For this review, take the finished solid that the model builds, in its own axes (mm). Coordinates: 2 decimals unless noted, no trailing zeros. Loops run counter-clockwise (first coordinate to the right, second up) from the corner with the lowest first, then second, coordinate; pieces in that order, holes last. Notation, with made-up numbers: M 65.25,18.25 L 99.25,18.25 A32 ccw 99.25,57.25 Z; hole C 58.5,44 d6. An arc over 180 degrees is marked long. Write each question's results on one line, items separated by ' | '. Start each with the question number.
```python
from build123d import *

# Parameters (mm, degrees)
F0_R     = 2
F1_DEPTH = 2


# Not quite as in the source:
# - a feature names something its author has since deleted; it is built from what else it names


with BuildPart() as f1:
    # F0 (on Top) → F1 (new body)
    with BuildSketch(Plane.XY):
        with BuildLine():
            Line((56.6317902379, -3.0349094544), (56.6317902379, 10.5057977874))
            ThreePointArc((56.6317902379, 10.5057977874), (57.9282334063, 11.0612910292), (58.8036425211, 9.955399302))
            Line((58.8036425211, 9.955399302), (58.8036425211, -3.3060063632))
            ThreePointArc((58.8036425211, -3.3060063632), (58.8059571474, -3.4285186947), (58.8128977225, -3.5508561677))
            Line((58.8128977225, -3.5508561677), (68.3904010917, -2.8257703951))
            ThreePointArc((68.3904010917, -2.8257703951), (69.9985927846, -2.4288509841), (71.3888536722, -1.5282954863))
            Line((71.3888536722, -1.5282954863), (71.9441100955, 13.8000454754))
            ThreePointArc((71.9441100955, 13.8000454754), (70.4479915869, 14.8624188349), (68.6693633039, 15.3135165823))
            Line((68.6693633039, 15.3135165823), (58.6544042145, 15.9537835574))
            Line((58.6544042145, 15.9537835574), (2.6067622363, 15.9537835574))
            ThreePointArc((2.6067622363, 15.9537835574), (0.4614561486, 15.0651686804), (-0.4271587284, 12.9198625927))
            Line((-0.4271587284, 12.9198625927), (-0.4271587284, -3.0349094544))
            Line((-0.4271587284, -3.0349094544), (3.8183579072, -3.0349094544))
            Line((3.8183579072, -3.0349094544), (3.8183579072, 2.3688513962))
            Line((3.8183579072, 2.3688513962), (3.8183579072, 10.5057977874))
            ThreePointArc((3.8183579072, 10.5057977874), (4.9481016159, 11.1006888991), (6.0778453246, 10.5057977874))
            Line((6.0778453246, 10.5057977874), (6.0778453246, 2.3688513962))
            Line((6.0778453246, 2.3688513962), (6.0778453246, -3.0349094544))
            ThreePointArc((6.0778453246, -3.0349094544), (6.9707155924, -3.9277797221), (7.8635858601, -3.0349094544))
            Line((7.8635858601, -3.0349094544), (7.8635858601, 2.3688513962))
            Line((7.8635858601, 2.3688513962), (7.8635858601, 10.5057977874))
            ThreePointArc((7.8635858601, 10.5057977874), (8.8748928484, 11.1003156957), (9.8861998366, 10.5057977874))
            Line((9.8861998366, 10.5057977874), (9.8861998366, 2.3688513962))
            Line((9.8861998366, 2.3688513962), (9.8861998366, -3.0349094544))
            ThreePointArc((9.8861998366, -3.0349094544), (10.8975068249, -4.0462164426), (11.9088138131, -3.0349094544))
            Line((11.9088138131, -3.0349094544), (11.9088138131, 2.3688513962))
            Line((11.9088138131, 2.3688513962), (11.9088138131, 10.5057977874))
            ThreePointArc((11.9088138131, 10.5057977874), (12.9201208014, 11.1003953408), (13.9314277896, 10.5057977874))
            Line((13.9314277896, 10.5057977874), (13.9314277896, 2.3688513962))
            Line((13.9314277896, 2.3688513962), (13.9314277896, -3.0349094544))
            ThreePointArc((13.9314277896, -3.0349094544), (14.9427347779, -4.0462164426), (15.9540417661, -3.0349094544))
            Line((15.9540417661, -3.0349094544), (15.9540417661, 2.3688513962))
            Line((15.9540417661, 2.3688513962), (15.9540417661, 10.5057977874))
            ThreePointArc((15.9540417661, 10.5057977874), (16.9653487543, 11.1012729968), (17.9766557426, 10.5057977874))
            Line((17.9766557426, 10.5057977874), (17.9766557426, -3.0349094544))
            Line((17.9766557426, -3.0349094544), (17.9766557426, -3.0600128507))
            ThreePointArc((17.9766557426, -3.0600128507), (18.987884836, -4.0587681408), (19.9991139294, -3.0600128507))
            Line((19.9991139294, -3.0600128507), (19.9991139294, -3.0349094544))
            Line((19.9991139294, -3.0349094544), (19.9991139294, 2.3688513962))
            Line((19.9991139294, 2.3688513962), (19.9991139294, 10.5057977874))
            ThreePointArc((19.9991139294, 10.5057977874), (21.0104988125, 11.0625593301), (22.0218836956, 10.5057977874))
            Line((22.0218836956, 10.5057977874), (22.0218836956, 2.3688513962))
            Line((22.0218836956, 2.3688513962), (22.0218836956, -3.0349094544))
            ThreePointArc((22.0218836956, -3.0349094544), (23.0331906838, -4.0270898738), (24.0444976721, -3.0349094544))
            Line((24.0444976721, -3.0349094544), (24.0444976721, 2.3688513962))
            Line((24.0444976721, 2.3688513962), (24.0444976721, 10.5057977874))
            ThreePointArc((24.0444976721, 10.5057977874), (25.0558046603, 11.1004906415), (26.0671116486, 10.5057977874))
            Line((26.0671116486, 10.5057977874), (26.0671116486, 2.3688513962))
            Line((26.0671116486, 2.3688513962), (26.0671116486, -3.0349094544))
            ThreePointArc((26.0671116486, -3.0349094544), (27.0784186368, -4.0282444578), (28.089725625, -3.0349094544))
            Line((28.089725625, -3.0349094544), (28.089725625, 2.3688513962))
            Line((28.089725625, 2.3688513962), (28.089725625, 10.5057977874))
            ThreePointArc((28.089725625, 10.5057977874), (29.1010326133, 11.1005861122), (30.1123396015, 10.5057977874))
            Line((30.1123396015, 10.5057977874), (30.1123396015, 2.3688513962))
            Line((30.1123396015, 2.3688513962), (30.1123396015, -3.0349094544))
            ThreePointArc((30.1123396015, -3.0349094544), (31.1236465898, -4.0401241658), (32.134953578, -3.0349094544))
            Line((32.134953578, -3.0349094544), (32.134953578, 2.3688513962))
            Line((32.134953578, 2.3688513962), (32.134953578, 10.5057977874))
            ThreePointArc((32.134953578, 10.5057977874), (33.1462605663, 11.0805944093), (34.1575675545, 10.5057977874))
            Line((34.1575675545, 10.5057977874), (34.1575675545, 2.3688513962))
            Line((34.1575675545, 2.3688513962), (34.1575675545, -3.0349094544))
            ThreePointArc((34.1575675545, -3.0349094544), (35.1688745428, -4.0284589293), (36.180181531, -3.0349094544))
            Line((36.180181531, -3.0349094544), (36.180181531, 2.3688513962))
            Line((36.180181531, 2.3688513962), (36.180181531, 10.5057977874))
            ThreePointArc((36.180181531, 10.5057977874), (37.1914885192, 11.0806196167), (38.2027955075, 10.5057977874))
            Line((38.2027955075, 10.5057977874), (38.2027955075, 2.3688513962))
            Line((38.2027955075, 2.3688513962), (38.2027955075, -3.0349094544))
            ThreePointArc((38.2027955075, -3.0349094544), (39.2141024957, -4.0246480782), (40.225409484, -3.0349094544))
            Line((40.225409484, -3.0349094544), (40.225409484, 2.3688513962))
            Line((40.225409484, 2.3688513962), (40.225409484, 10.5057977874))
            ThreePointArc((40.225409484, 10.5057977874), (41.2367164722, 11.0799992786), (42.2480234605, 10.5057977874))
            Line((42.2480234605, 10.5057977874), (42.2480234605, 2.3688513962))
            Line((42.2480234605, 2.3688513962), (42.2480234605, -3.0349094544))
            ThreePointArc((42.2480234605, -3.0349094544), (43.2593304487, -4.0462164426), (44.270637437, -3.0349094544))
            Line((44.270637437, -3.0349094544), (44.270637437, 2.3688513962))
            Line((44.270637437, 2.3688513962), (44.270637437, 10.5057977874))
            ThreePointArc((44.270637437, 10.5057977874), (45.2819444252, 11.0763000676), (46.2932514135, 10.5057977874))
            Line((46.2932514135, 10.5057977874), (46.2932514135, 2.3688513962))
            Line((46.2932514135, 2.3688513962), (46.2932514135, -3.0349094544))
            ThreePointArc((46.2932514135, -3.0349094544), (47.3045584017, -4.0362897846), (48.3158653899, -3.0349094544))
            Line((48.3158653899, -3.0349094544), (48.3158653899, 2.3688513962))
            Line((48.3158653899, 2.3688513962), (48.3158653899, 10.5057977874))
            ThreePointArc((48.3158653899, 10.5057977874), (49.3271723782, 11.0768378201), (50.3384793664, 10.5057977874))
            Line((50.3384793664, 10.5057977874), (50.3384793664, 2.3688513962))
            Line((50.3384793664, 2.3688513962), (50.3384793664, -3.0349094544))
            ThreePointArc((50.3384793664, -3.0349094544), (51.3497863547, -4.0273604844), (52.3610933429, -3.0349094544))
            Line((52.3610933429, -3.0349094544), (52.3610933429, 2.3688513962))
            Line((52.3610933429, 2.3688513962), (52.3610933429, 10.5057977874))
            ThreePointArc((52.3610933429, 10.5057977874), (53.4851541573, 11.0994017223), (54.6092149717, 10.5057977874))
            Line((54.6092149717, 10.5057977874), (54.6092149717, 2.3688513962))
            Line((54.6092149717, 2.3688513962), (54.6092149717, -3.0349094544))
            ThreePointArc((54.6092149717, -3.0349094544), (55.6205026048, -4.039959639), (56.6317902379, -3.0349094544))
        make_face()
        with Locations((68.012945354, 2.1599619649)):
            Circle(F0_R, mode=Mode.SUBTRACT)
        with Locations((68.3503592405, 10.3237033185)):
            Circle(F0_R, mode=Mode.SUBTRACT)
    extrude(amount=F1_DEPTH)


solid = f1.part
```
Q1. Take a section at C-C, the plane x = 37.5. Give the boundary of the cut face in (y, z), then the cut area to 3 significant figures.
Q2. The part is to be moulded in two halves that separate along X. For faces 1 (the face through (35, 6, 0)), 2 (the face through (11.909, 4, 1)), say which applies: pulls with the +X half, pulls with the -X half, needs draft (parallel to the pull), parting line crosses it, or undercut.
Q3. To check wall thickness, follow line 1 along Y through (x, z) = (51.5, 1.15); line 2 along Y through (x, z) = (45.5, 1.4); line 3 along X through (y, z) = (11.25, 0.25). State the ranges of each line that lie inside material, in increasing order.
Q4. Insertion check: P1, Ø0.6, axis at y = 6, z = 1, coming from the +X side; P2, Ø10, axis at x = 8, y = 2, coming from the -Z side. Each pin has a flat end and moves straight along its axis. Give the tip position at first contact, or say it passes through.
Q5. Take a section at A-A, the plane y = 7.5. Give the number of separate pieces and of enclosed holes in the cut face, then the cut area to 3 significant figures.
Results:
1) outline: M 11.04,0 L 15.95,0 L 15.95,2 L 11.04,2 Z | area: 9.83 mm^2
2) face 1: needs draft | face 2: undercut
3) line 1: -4.02 to 15.95 | line 2: 11.06 to 15.95 | line 3: -0.43 to 66.58, 70.12 to 71.85
4) P1: x = 71.67 | P2: z = 0
5) separate pieces: 15 | enclosed holes: 0 | area: 86.4 mm^2
